Verification items for the finished model (mm, model axes). A direction names the side the tool comes from. Give positions to 0.01 mm unless a question says otherwise; leave off trailing zeros. Loops run counter-clockwise (first coordinate to the right, second up) from the corner with the lowest first, then second, coordinate; pieces in that order, holes last. Notation, with made-up numbers: (12.5, -6.5) - (59.5, -6.5) arc R17 ccw to (59.5, 10.5) - close; hole circle Ø2 at (28.25, 63.25). An arc over 180 degrees is marked (long way). One line per item, written item: value. Start each with the question number.
1. Mould release check, pull along Y, two halves, no side actions. Record for faces 1 (the cylindrical face through (-21.586, 0.208, 26.451)), 2 (the flat face through (27, 0, 0)), 3 (the cylindrical face through (0.511, 27.495, 18.543)), 4 (the cylindrical face through (28.615, -9.011, 18.123)): pulls with the +Y half, pulls with the -Y half, needs draft (parallel to the pull), parting line crosses it, or undercut.
2. Access from +Z, -Z, +X, -X, +Y, -Y to the whole of each face (thin tool, end or side, straight path). Record for faces 5 (the cylindrical face through (12.205, -0.867, 25.028)), 6 (the flat face through (-28, 0, 0)), 7 (the flat face through (0, -6.658, 25)).
3. Scan lines: L1, parallel to Y at x = -8.3, z = 24.3; L2, parallel to Y at x = 6.5, z = 28; L3, parallel to Y at x = 4, z = 25.5. Record each from-to range of solid material in increasing order. Write a range as [from, to].
4. Sectioned sample at D-D (y = 0). Count the separate pieces of the cut face and the enclosed holes in it, plus the area to 3 significant figures.
5. Sectioned sample at A-A (x = 0). Record the cut outline in (y, z).
6. Sectioned sample at B-B (z = 5.5). Record the cut outline in (x, y).
7. Gauge pin test, flat ends, axial feed: pin 1 (1.5 mm diameter, centred on y = -14.5, z = 16, fed in from +X); pin 2 (1.6 mm diameter, centred on x = 8.3, y = 0, fed in from +Z); pin 3 (5 mm diameter, centred on x = -20, y = 0, fed in from -Z); pin 4 (1.5 mm diameter, centred on x = -13.5, z = 14, fed in from -Y). Record the tip position at first contact, or that the pin passes through.
8. Sectioned sample at C-C (y = 9.5). Record the cut outline in (x, z), plus the area to 3 significant figures.
Autodesk Inventor part; units mm, degrees
ref_plane "YZ Plane" through (0, 0, 0) normal (1, 0, 0) x (0, 1, 0)
ref_plane "XZ Plane" through (0, 0, 0) normal (0, 1, 0) x (-1, 0, 0)
ref_plane "XY Plane" through (0, 0, 0) normal (0, 0, 1) x (1, 0, 0)
sketch "スケッチ1" plane through (0, 0, 0) normal (0, 0, 1) x (1, 0, 0)
  circle A0 centre (0, 0) radius 30
  dimension "d0" = 60
extrude "押し出し1" add sketch "スケッチ1" along normal blind 30
sketch "スケッチ2" plane through (0, 0, 30) normal (0, 0, 1) x (1, 0, 0)
  circle A0 centre (0, 0) radius 26
  dimension "d3" = 52
extrude "押し出し2" cut sketch "スケッチ2" against normal blind 50
sketch "スケッチ3" plane through (0, 0, 0) normal (0, 0, 1) x (1, 0, 0)
  point P0 (0, 0)
sketch "スケッチ4" plane through (0, 0, 0) normal (1, 0, 0) x (0, 1, 0)
  line L0 (30, 0) -> (-30, 0)
  line L1 (-30, 0) -> (-30, 30)
  arc A0 (30, 0) -> (-30, 0) centre (0, 0) ccw
  dimension "d6" = 30
extrude "押し出し3" cut sketch "スケッチ4" along normal mid plane 50
sketch "スケッチ5" plane through (0, 0, 30) normal (0, 0, 1) x (1, 0, 0)
  circle A0 centre (0, 0) radius 27.5
extrude "押し出し4" add sketch "スケッチ5" against normal blind 7
sketch "スケッチ19" plane through (0, 0, 30) normal (0, 0, 1) x (1, 0, 0)
  circle A0 centre (0, 0) radius 27.5
  line L0 (27.5, -6.6575) -> (-27.5, -6.6575)
  line L1 (-27.5, -6.6575) -> (-27.5, 6.6575)
  line L2 (-27.5, 6.6575) -> (27.5, 6.6575)
  line L3 (27.5, 6.6575) -> (27.5, -6.6575)
  line L4 (27.5, -6.6575) -> (-27.5, 6.6575) construction
  line L5 (-27.5, -6.6575) -> (27.5, 6.6575) construction
  point P0 (26.682, -6.6575)
  point P1 (-26.682, -6.6575)
  point P2 (-26.682, 6.6575)
  point P3 (26.682, 6.6575)
extrude "押し出し11" cut sketch "スケッチ19" against normal blind 60 contours L2 A0 | A0 L0
sketch "スケッチ22" plane through (0, 0, 30) normal (0, 0, 1) x (1, 0, 0)
  point P0 (0, 0)
sketch "スケッチ23" plane through (0, 0, 30) normal (0, 0, 1) x (1, 0, 0)
  point P0 (0, 0)
  point P1 (-20, 0)
  point P2 (20, 0)
  dimension "d67" = 20
  dimension "d68" = 20
hole "穴4" at (-20, 0, 30) at (20, 0, 30) direction (0, 0, -1) diameter 3.2 depth 8.8 tip angle 118
sketch "スケッチ25" plane through (0, 0, 30) normal (0, 0, 1) x (1, 0, 0)
  point P0 (0, 0)
  point P1 (0, 0)
hole "穴5" at (0, 0, 30) direction (0, 0, -1) diameter 1.5 depth 8.8 tip angle 118
sketch "スケッチ27" plane through (0, 0, 23) normal (0, 0, -1) x (-1, 0, 0)
  point P0 (0, 0)
  point P1 (8.3, 0)
  point P2 (-8.3, 0)
  dimension "d95" = 8.3
  dimension "d96" = 8.3
hole "穴7" at (-8.3, 0, 23) at (8.3, 0, 23) direction (0, 0, 1) diameter 1.8 depth 8.8 tip angle 118 counterbore diameter 8 counterbore depth 4
properties part number "20220527_仮筒"
Results are:
1. face 1: undercut
1. face 2: needs draft
1. face 3: undercut
1. face 4: parting line crosses it
2. face 5: -Z
2. face 6: -Z, +X, -X, +Y, -Y
2. face 7: +Z, -Z
3. L1: y = [-28.83, -26.22], [-6.66, -4], [4, 6.66], [26.22, 28.83]
3. L2: y = [-29.29, -26.72], [-6.66, 6.66], [26.72, 29.29]
3. L3: y = [-29.73, -27.21], [-6.66, 6.66], [27.21, 29.73]
4. separate pieces: 6
4. enclosed holes: 0
4. area: 474 mm^2
5. outline: (-30, 0) arc R30 cw to (-27.5, 11.99) - (-27.5, 30) - (-30, 30) - close; (-6.66, 23) - (-0.75, 23) - (-0.75, 30) - (-6.66, 30) - close; (0.75, 23) - (6.66, 23) - (6.66, 30) - (0.75, 30) - close; (27.5, 11.99) arc R30 cw to (30, 0) - (30, 30) - (27.5, 30) - close
6. outline: (-26.68, -6.66) - (-25.13, -6.66) arc R26 cw to (-25.13, 6.66) - (-26.68, 6.66) arc R27.5 cw to (-25, 11.46) - (-25, 16.58) arc R30 ccw to (-25, -16.58) - (-25, -11.46) arc R27.5 cw to start; (-5.5, -29.49) arc R30 ccw to (5.5, -29.49) - close; (-5.5, 29.49) - (5.5, 29.49) arc R30 ccw to start; (25, -16.58) arc R30 ccw to (25, 16.58) - (25, 11.46) arc R27.5 cw to (26.68, 6.66) - (25.13, 6.66) arc R26 cw to (25.13, -6.66) - (26.68, -6.66) arc R27.5 cw to (25, -11.46) - close
7. pin 1: stops at x = 26.66
7. pin 2: passes through
7. pin 3: stops at z = 23
7. pin 4: stops at y = -27.16
8. outline: (-28.46, 0) - (-25.81, 0) - (-25.81, 30) - (-28.46, 30) - close; (25.81, 0) - (28.46, 0) - (28.46, 30) - (25.81, 30) - close
8. area: 159 mm^2
